```python
from build123d import *

# Parameters (mm, degrees)
SKETCH2_R           = 8
BOSS_EXTRUDE1_DEPTH = 30
BOSS_EXTRUDE3_DEPTH = 10
BOSS_EXTRUDE4_DEPTH = 7
FILLET1_R           = 0.4
SKETCH12_R          = 1.1
SKETCH12_R_2        = 1.75
CUT_EXTRUDE2_DEPTH  = 42.569219478
SKETCH13_R          = 1.7
CUT_EXTRUDE3_DEPTH  = 43.12296985


with BuildPart() as part:
    # Sketch2 → Boss-Extrude1 (new body)
    with BuildSketch(Plane(origin=(0, 0, 0), x_dir=(1, 0, 0), z_dir=(0, 1, 0))):
        with Locations(Location((0, 0, 0), (0, 0, 270))):
            Circle(SKETCH2_R)
    extrude(amount=BOSS_EXTRUDE1_DEPTH)

    # Sketch4 → Boss-Extrude3 (add)
    with BuildSketch(Plane(origin=(0, 30, 0), x_dir=(1, 0, 0), z_dir=(0, 1, 0))):
        with BuildLine():
            Line((2.504502892, -1.8), (2.504502892, 1.8))
            ThreePointArc((2.504502892, 1.8), (0, 3.30267653), (-2.504502892, 1.8))
            Line((-2.504502892, 1.8), (-2.504502892, -1.8))
            ThreePointArc((-2.504502892, -1.8), (0, -3.30267653), (2.504502892, -1.8))
        make_face()
    boss_extrude3 = extrude(amount=BOSS_EXTRUDE3_DEPTH)

    # Sketch8 → Boss-Extrude4 (add)
    with BuildSketch(Plane(origin=(0, 30, 0), x_dir=(1, 0, 0), z_dir=(0, 1, 0))):
        with BuildLine():
            Line((-1.2, -3.84404132), (1.2, -3.84404132))
            ThreePointArc((1.2, -3.84404132), (1.803521194, -4.169699523), (2, -4.826728575))
            Line((2, -4.826728575), (-2, -4.826728575))
            ThreePointArc((-2, -4.826728575), (-1.803521194, -4.169699523), (-1.2, -3.84404132))
        make_face()
    extrude(amount=BOSS_EXTRUDE4_DEPTH)

    # Fillet1
    fillet1_edges = [part.edges().sort_by_distance(p)[0] for p in [
        (0, 30, 4.826728575),
        (0, 30, -3.30267653),
        (0, 30, 3.30267653),
    ]]
    fillet(fillet1_edges, radius=FILLET1_R)

    # Sketch12 → Cut-Extrude2 (cut, through all)
    with BuildSketch(Plane(origin=(0, 0, 0), x_dir=(1, 0, 0), z_dir=(0, 1, 0))):
        with Locations(Location((0, 5.887857779, 0), (0, 0, 270))):
            Circle(SKETCH12_R)
        with Locations(Location((4.511323968, -3.260456868, 0), (0, 0, 270))):
            Circle(SKETCH12_R_2)
    extrude(amount=CUT_EXTRUDE2_DEPTH, mode=Mode.SUBTRACT)

    # Sketch13 → Cut-Extrude3 (cut, through all)
    with BuildSketch(Plane.ZY.offset(2.504502892)):
        with Locations((0, 37.692003777)):
            Circle(SKETCH13_R)
    cut_extrude3 = extrude(amount=-CUT_EXTRUDE3_DEPTH, mode=Mode.SUBTRACT)

    # Mirror1: Boss-Extrude3, Cut-Extrude3 across plane
    add(boss_extrude3.mirror(Plane.ZX.offset(15)))
    add(cut_extrude3.mirror(Plane.ZX.offset(15)), mode=Mode.SUBTRACT)


solid = part.part
```
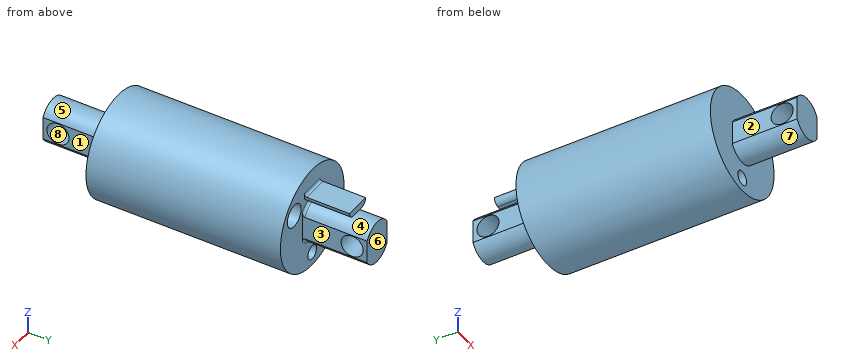
Build history of the part. All positions in model axes, mm. Face numbers are marked on the shaded views. A direction names the side the tool comes from. Round coordinates to 2 decimals unless told otherwise and drop trailing zeros. Order: outer loops, then holes, each group sorted by start corner. A loop starts at its lowest first (then second) coordinate and runs counter-clockwise, first axis right, second up. Notation, with made-up numbers: (15.5, 89) - (73.5, 89) arc R7 cw to (73.5, 93) - close; hole circle Ø8 at (-17, 1.5). An arc over 180 degrees is marked (long way). Use a Markdown table: item, result.
1) Pull direction Z, two halves, no side cores. Call the marked faces 6, 7 and 8: pulls with the +Z half, pulls with the -Z half, needs draft (parallel to the pull), parting line crosses it, or undercut.
Recorded:
| item | result |
|---|---|
| face 6 | needs draft |
| face 7 | pulls with the -Z half |
| face 8 | undercut |
2) Saw through at A-A on y = 34. Write the cut outline in (x, z).
Recorded:
| item | result |
|---|---|
| outline | (-2.5, -1.8) arc R2.84 ccw to (2.5, -1.8) - (2.5, 1.8) arc R2.84 ccw to (-2.5, 1.8) - close; (-2, 4.83) arc R0.9 ccw to (-1.2, 3.84) - (1.2, 3.84) arc R0.9 ccw to (2, 4.83) - close |
3) Saw through at B-B on z = 0. Write the cut outline in (x, y), and give its area (3 significant figures).
Recorded:
| item | result |
|---|---|
| outline | (-8, 0) - (-2.5, 0) - (-2.5, -5.99) - (2.5, -5.99) - (2.5, 0) - (8, 0) - (8, 30) - (2.5, 30) - (2.5, 35.99) - (-2.5, 35.99) - (-2.5, 30) - (-8, 30) - close; (-2.5, -10) - (2.5, -10) - (2.5, -9.39) - (-2.5, -9.39) - close; (-2.5, 39.39) - (2.5, 39.39) - (2.5, 40) - (-2.5, 40) - close |
| area | 546 mm² |
4) Wall check: L1, parallel to Y at x = 0.5, z = 0; L2, parallel to Z at x = 0, y = 32.5; L3, parallel to Y at x = -3.75, z = -1.75. Give the ranges that are in metal, low to high.
Recorded:
| item | result |
|---|---|
| L1 | y = -10 to -9.39, -5.99 to 35.99, 39.39 to 40 |
| L2 | z = -3.3 to 3.3, 3.84 to 4.83 |
| L3 | y = 0 to 30 |
5) Saw through at C-C on x = 0. Write the cut outline in (y, z), and give its area (3 significant figures).
Recorded:
| item | result |
|---|---|
| outline | (-10, -3.3) - (0, -3.3) - (0, -4.79) - (30, -4.79) - (30, -3.7) arc R0.4 cw to (30.4, -3.3) - (40, -3.3) - (40, 3.3) - (30.4, 3.3) arc R0.4 cw to (30, 3.7) - (30, 3.84) - (37, 3.84) - (37, 4.83) - (30.4, 4.83) arc R0.4 cw to (30, 5.23) - (30, 8) - (0, 8) - (0, 3.3) - (-10, 3.3) - close; (0, -8) - (30, -8) - (30, -6.99) - (0, -6.99) - close; hole circle Ø3.4 at (-7.69, 0); hole circle Ø3.4 at (37.69, 0) |
| area | 535 mm² |
6) Flat gauge pins, fed straight in: pin 1 Ø8 at (y, z) = (12.5, 6) entering from +X; pin 2 Ø4 at (y, z) = (35.5, 0.5) entering from +X; pin 3 Ø1.2 at (x, y) = (-0.5, 34) entering from +Z. Where does each tip first touch, or does it go through?
Recorded:
| item | result |
|---|---|
| pin 1 | stops at x = 7.75 |
| pin 2 | stops at x = 2.5 |
| pin 3 | stops at z = 4.83 |
7) Tool access for the marked faces 1, 2, 3, 4 and 5: list every direction of +Z, -Z, +X, -X, +Y, -Y with a clear straight run to the whole face (end or side of a thin tool).
Recorded:
| item | result |
|---|---|
| face 1 | +Z, -Z, +X, -Y |
| face 2 | +Z, -Z, -X, -Y |
| face 3 | +Z, -Z, +X, +Y |
| face 4 | +Y |
| face 5 | +Z, -Y |
8) Saw through at D-D on y = -4. Write the cut outline in (x, z).
Recorded:
| item | result |
|---|---|
| outline | (-2.5, -1.8) arc R2.84 ccw to (2.5, -1.8) - (2.5, 1.8) arc R2.84 ccw to (-2.5, 1.8) - close |
